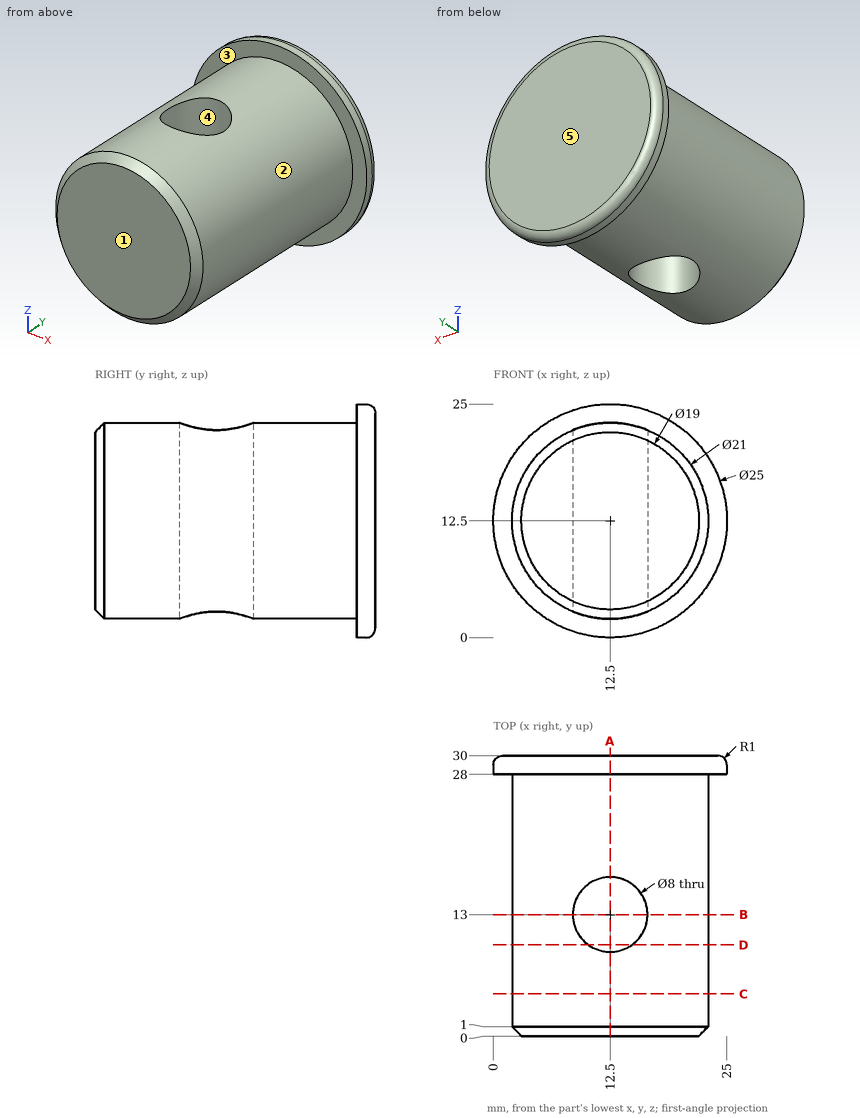
Verification items for this drawing (mm, ordinates from the low corner). A direction names the side the tool comes from. Coordinates: 2 decimals unless noted, no trailing zeros. Loops run counter-clockwise (first coordinate to the right, second up) from the corner with the lowest first, then second, coordinate; pieces in that order, holes last. Notation, with made-up numbers: (-18.5, 79) -> (35.5, 79) arc R19 cw to (35.5, 112) -> close; hole circle Ø4 at (1.25, 48). An arc over 180 degrees is marked (long way). Answer in a Markdown table with one row per item. Add a question column.
1. Section check C-C, the plane y = 4.5. Enter the section's corners in (x, z), then the cut area to 3 significant figures.
2. Access from +Z, -Z, +X, -X, +Y, -Y to the whole of each face (thin tool, end or side, straight path). Record for the marked faces 1 and 2.
3. Section check D-D, the plane y = 9.75. Enter the section's corners in (x, z), then the cut area to 3 significant figures.
4. Section check B-B, the plane y = 13. Enter the section's corners in (x, z).
5. Draft check along Y on the marked faces 3, 4 and 5. Enter one of: +Y half, -Y half, draft (parallel to the pull), parting line (faces both ways), or undercut.
6. Material ranges on probe 1 along X at (y, z) = (13, 12.5); probe 2 along X at (y, z) = (9.75, 6); probe 3 along Y at (x, z) = (4.25, 5), recorded low to high. Write a range as [from, to].
7. Section check A-A, the plane x = 12.5. Enter the section's corners in (y, z).
8. Depth check by flat-ended pin: P1, Ø6, axis at x = 5.5, y = 6, coming from the +Z side; P2, Ø3, axis at x = 16.5, y = 9, coming from the -Z side; P3, Ø13, axis at x = 12.5, y = 13, coming from the +Z side. Enter the tip coordinate at first touch or a pass-through.
Derived:
| question | item | result |
|---|---|---|
| 1 | outline | circle Ø21 at (12.5, 12.5) |
| 1 | area | 346 mm² |
| 2 | face 1 | +Z, -Z, +X, -X, -Y |
| 2 | face 2 | -Y |
| 3 | outline | (10.17, 2.26) -> (10.17, 22.74) arc R10.5 ccw to start; (14.83, 2.26) arc R10.5 ccw to (14.83, 22.74) -> close |
| 3 | area | 249 mm² |
| 4 | outline | (8.5, 2.79) -> (8.5, 22.21) arc R10.5 ccw to start; (16.5, 2.79) arc R10.5 ccw to (16.5, 22.21) -> close |
| 5 | face 3 | -Y half |
| 5 | face 4 | undercut |
| 5 | face 5 | +Y half |
| 6 | probe 1 | x = [2, 8.5], [16.5, 23] |
| 6 | probe 2 | x = [4.25, 10.17], [14.83, 20.75] |
| 6 | probe 3 | y = [28, 30] |
| 7 | outline | (0, 3) -> (1, 2) -> (9, 2) -> (9, 23) -> (1, 23) -> (0, 22) -> close; (17, 2) -> (28, 2) -> (28, 0) -> (29, 0) arc R1 ccw to (30, 1) -> (30, 24) arc R1 ccw to (29, 25) -> (28, 25) -> (28, 23) -> (17, 23) -> close |
| 8 | P1 | stops at z = 22.21 |
| 8 | P2 | stops at z = 2.3 |
| 8 | P3 | stops at z = 23 |
